Part model, mm, in its own coordinate system. Face numbers are marked on the shaded views. A direction names the side the tool comes from. Round coordinates to 2 decimals unless told otherwise and drop trailing zeros. Order: outer loops, then holes, each group sorted by start corner. A loop starts at its lowest first (then second) coordinate and runs counter-clockwise, first axis right, second up. Notation, with made-up numbers: (-13, 82.25) - (7, 82.25) arc R19 cw to (7, 98.25) - close; hole circle Ø2 at (-33, 55). An arc over 180 degrees is marked (long way). Return JSON: item names as keys, results as strings. Group by question number.
Item 1: Probe probe 1 along Z at (x, y) = (4.25, 0.3); probe 2 along X at (y, z) = (3.5, -0.5); probe 3 along Y at (x, z) = (1.5, -4.5). List the from-to ranges inside material, lowest first.
Item 2: Saw through at C-C on y = 0.5. List the corners of the cut face in (x, z), and give its area (3 significant figures).
Item 3: Drop flat-ended pins along their axis: pin 1 (5 mm diameter, centred on x = 4.25, z = -5.75, fed in from +Y); pin 2 (4 mm diameter, centred on x = -2, y = 7, fed in from +Z); pin 3 (1.5 mm diameter, centred on y = 6, z = 0.5, fed in from +X); pin 4 (0.8 mm diameter, centred on x = -4.5, y = 8.5, fed in from +Z). Give the stop position or say it passes through.
Item 4: Saw through at B-B on x = 4.25. List the corners of the cut face in (y, z).
Item 5: Tool access for the marked faces 1, 2 and 3: list every direction of +Z, -Z, +X, -X, +Y, -Y with a clear straight run to the whole face (end or side of a thin tool).
Item 6: Saw through at A-A on z = 5.75. List the corners of the cut face in (x, y).
Item 7: Saw through at D-D on z = -2. List the corners of the cut face in (x, y).
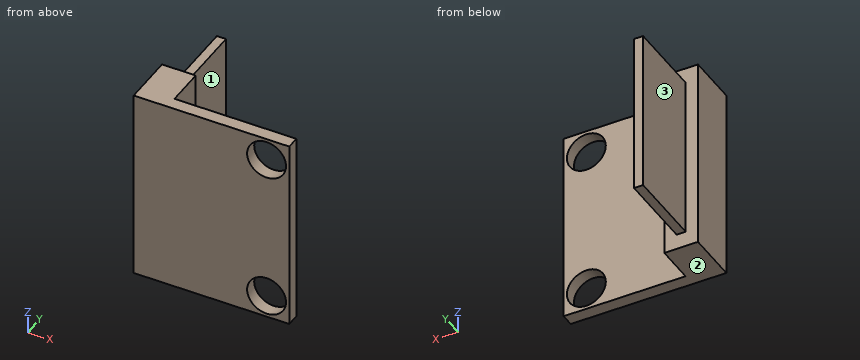
Autodesk Inventor part; units mm, degrees
ref_plane "YZ Plane" through (0, 0, 0) normal (1, 0, 0) x (0, 1, 0)
ref_plane "XZ Plane" through (0, 0, 0) normal (0, 1, 0) x (-1, 0, 0)
ref_plane "XY Plane" through (0, 0, 0) normal (0, 0, 1) x (1, 0, 0)
sketch "Sketch1" plane through (0, 0, 0) normal (0, 1, 0) x (-1, 0, 0)
  line L0 (-6, 7.5) -> (6, 7.5)
  line L1 (6, 7.5) -> (6, -7.5)
  line L2 (6, -7.5) -> (-6, -7.5)
  line L3 (-6, -7.5) -> (-6, 7.5)
  line L4 (-6, 7.5) -> (6, -7.5) construction
  line L5 (6, 7.5) -> (-6, -7.5) construction
  line L6 (-6, 7.5) -> (-4.25, 7.5)
  line L7 (-6, 5.75) -> (-6, 7.5)
  circle A0 centre (-4.25, 5.75) radius 1.5
  line L8 (0, 0) -> (-1.7804, 0)
  circle A1 centre (-4.25, -5.75) radius 1.5
  dimension "d0" = 12
  dimension "d1" = 15
  dimension "d4" = 3
  dimension "d7" = 1.75
extrude "Extrusion1" add sketch "Sketch1" along normal blind 1
sketch "Sketch2" plane through (0, 1, 0) normal (0, 1, 0) x (1, 0, 0)
  line L0 (-6, 7.5) -> (-6, -7.5)
  line L1 (-3.4, 7.5) -> (-6, 7.5)
  line L2 (-6, 7.5) -> (-6, -7.5)
  line L3 (-6, -7.5) -> (-3.4, -7.5)
  line L4 (-3.4, -7.5) -> (-3.4, 7.5)
  line L5 (-3.4, 7.5) -> (-6, -7.5) construction
  line L6 (-6, 7.5) -> (-3.4, -7.5) construction
  point P0 (0, 0)
  dimension "d9" = 2.6
  dimension "d10" = 15
extrude "Extrusion2" add sketch "Sketch2" along normal blind 3
sketch "Sketch3" plane through (0, 4, 0) normal (0, 1, 0) x (1, 0, 0)
  line L0 (-6, -7.5) -> (-6, -8)
  line L1 (6, 7.5) -> (-3.4, 7.5)
  line L2 (-6, 7.5) -> (-6, -7.5)
  line L3 (-3.4, -7.5) -> (-3.4, 7.5)
  line L4 (-4.35, -6.3) -> (-5.05, -6.3)
  line L5 (-5.05, -6.3) -> (-5.05, 6.3)
  line L6 (-5.05, 6.3) -> (-4.35, 6.3)
  line L7 (-4.35, 6.3) -> (-4.35, -6.3)
  line L8 (-4.35, -6.3) -> (-5.05, 6.3) construction
  line L9 (-5.05, -6.3) -> (-4.35, 6.3) construction
  point P0 (0, 0)
  point P1 (-4.7, 0)
  dimension "d13" = 12.6
  dimension "d14" = 0.7
extrude "Extrusion3" add sketch "Sketch3" along normal blind 6
properties part number "SensorPresionHumedadTemp"
Filled in:
{
 "1": {"probe 1": "z = -7.5 to -7.25, -4.25 to 4.25, 7.25 to 7.5", "probe 2": "x = -6 to -3.4", "probe 3": "y = 0 to 1"},
 "2": {"outline": "(-6, -7.5) - (6, -7.5) - (6, 7.5) - (-6, 7.5) - close; hole circle Ø3 at (4.25, -5.75); hole circle Ø3 at (4.25, 5.75)", "area": "166 mm^2"},
 "3": {"pin 1": "stops at y = 1", "pin 2": "passes through", "pin 3": "stops at x = -4.35", "pin 4": "stops at z = 6.3"},
 "4": {"outline": "(0, -7.5) - (1, -7.5) - (1, -7.25) - (0, -7.25) - close; (0, -4.25) - (1, -4.25) - (1, 4.25) - (0, 4.25) - close; (0, 7.25) - (1, 7.25) - (1, 7.5) - (0, 7.5) - close"},
 "5": {"face 1": "+Z, -Z, +X, +Y", "face 2": "-Z, +X, -X, +Y, -Y", "face 3": "+Z, -Z, -X, +Y"},
 "6": {"outline": "(-6, 0) - (2.75, 0) - (2.75, 1) - (-3.4, 1) - (-3.4, 4) - (-4.35, 4) - (-4.35, 10) - (-5.05, 10) - (-5.05, 4) - (-6, 4) - close; (5.75, 0) - (6, 0) - (6, 1) - (5.75, 1) - close"},
 "7": {"outline": "(-6, 0) - (6, 0) - (6, 1) - (-3.4, 1) - (-3.4, 4) - (-4.35, 4) - (-4.35, 10) - (-5.05, 10) - (-5.05, 4) - (-6, 4) - close"}
}
